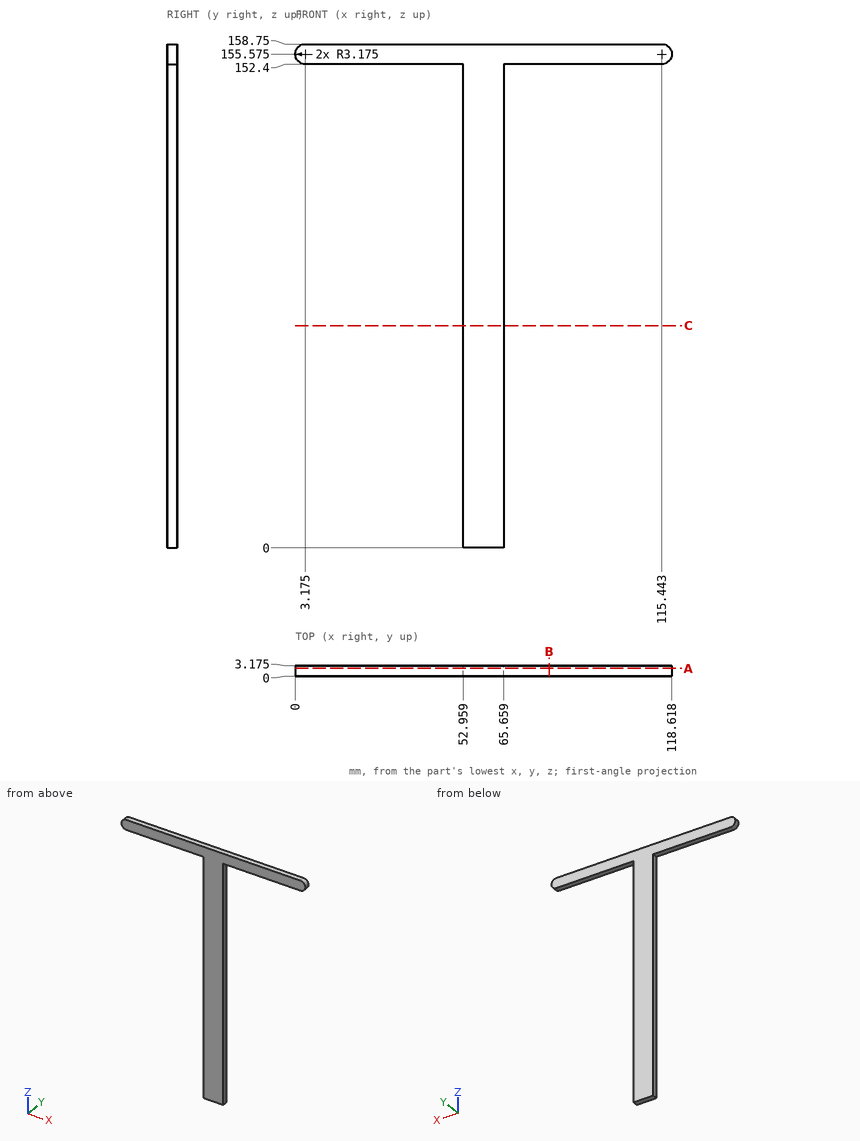
Source: three-view drawing plus pictorial views. Frame: mm from the lowest corner of the part. Coordinates: 2 decimals unless noted, no trailing zeros. Write each loop counter-clockwise with the first axis right and the second up, starting at its lowest first coordinate (ties: lowest second). Pieces come first, ordered by that corner, then holes. Notation, with made-up numbers: (28.25, 86) - (68.25, 86) arc R32 ccw to (68.25, 116) - close; hole circle Ø5 at (39, 10). An arc over 180 degrees is marked (long way). Return JSON: item names as keys, results as strings.
Item 1: Section query A-A (y = 2.4). Output: boundary loops of the cut face in (x, z) (3 decimals).
Completed:
{"outline": "(3.175, 152.4) - (52.959, 152.4) - (52.959, 0) - (65.659, 0) - (65.659, 152.4) - (115.443, 152.4) arc R3.175 ccw to (115.443, 158.75) - (3.175, 158.75) arc R3.175 ccw to start"}
Item 2: Section query C-C (z = 70). Output: boundary loops of the cut face in (x, y) (3 decimals).
Completed:
{"outline": "(52.959, 0) - (65.659, 0) - (65.659, 3.175) - (52.959, 3.175) - close"}
Item 3: Line query: L1, parallel to Z at x = 39.5, y = 2; L2, parallel to X at y = 1.25, z = 49. Output: solid intervals per line, ascending.
Completed:
{"L1": "z = 152.4 to 158.75", "L2": "x = 52.96 to 65.66"}
Item 4: Section query B-B (x = 80). Output: boundary loops of the cut face in (y, z) (3 decimals), and give its area (3 significant figures).
Completed:
{"outline": "(0, 152.4) - (3.175, 152.4) - (3.175, 158.75) - (0, 158.75) - close", "area": "20.2 mm2"}
Item 5: Pin query (flat end, axial travel): pin 1 Ø1.6 at (x, y) = (82, 2.5) entering from -Z. Return the tip coordinate at first contact, or that it passes through.
Completed:
{"pin 1": "stops at z = 152.4"}
